Answer from the drawing. Dimensions are ordinates in mm from the lowest x, y and z of the part. Give positions to 0.01 mm unless a question says otherwise; leave off trailing zeros. Write each loop counter-clockwise with the first axis right and the second up, starting at its lowest first coordinate (ties: lowest second). Pieces come first, ordered by that corner, then holes. Notation, with made-up numbers: M -16.5,-15.75 L 0.5,-15.75 A28 cw 0.5,5.25 Z; hole C -13,83 d6. An arc over 180 degrees is marked long. Write each question's results on one line, items separated by ' | '. Start each with the question number.
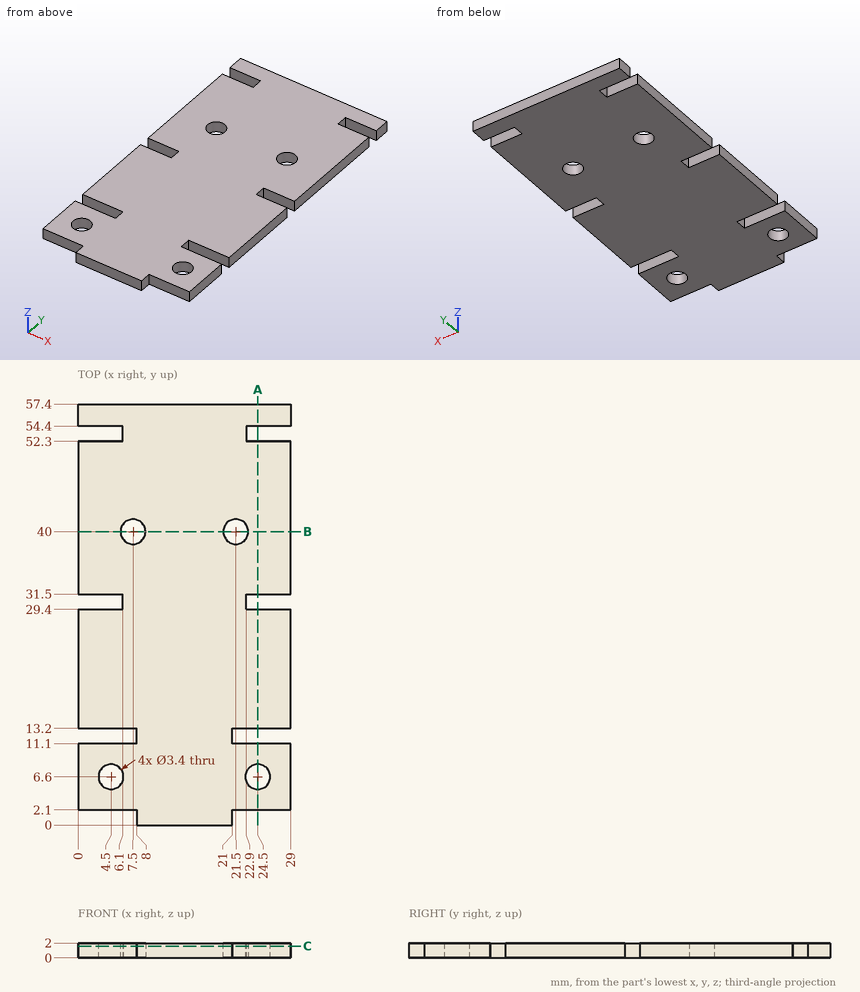
Item 1: Section C-C, the plane z = 1.6 is taken. Give the number of separate pieces and of enclosed holes in the cut face, then the cut area to 3 significant figures.
Item 2: Section B-B, the plane y = 40 is taken. Determine the outline of the cut face in (x, z).
Item 3: Straight lines are drawn through the part: line 1 (Y direction, x = 26.5, z = 1.4); line 2 (Y direction, x = 4.5, z = 0.5); line 3 (Y direction, x = 7.5, z = 1.4). For each, find the intervals that lie inside material, in ascending order.
Item 4: Section A-A, the plane x = 24.5 is taken. Determine the outline of the cut face in (y, z).
Item 5: Given P1, Ø2, axis at x = 4.5, y = 6.6, coming from the -Z side; P2, Ø1, axis at y = 53, z = 1, coming from the -X side; P3, Ø1, axis at x = 23.5, z = 1, coming from the -Y side, each flat-ended and moving along its own axis, determine where each tip first touches the part or whether it passes through.
Worked out:
1) separate pieces: 1 | enclosed holes: 4 | area: 1,510 mm²
2) outline: M 0,0 L 5.8,0 L 5.8,2 L 0,2 Z; M 9.2,0 L 19.8,0 L 19.8,2 L 9.2,2 Z; M 23.2,0 L 29,0 L 29,2 L 23.2,2 Z
3) line 1: y = 2.1 to 11.1, 13.2 to 29.4, 31.5 to 52.3, 54.4 to 57.4 | line 2: y = 2.1 to 4.9, 8.3 to 11.1, 13.2 to 29.4, 31.5 to 52.3, 54.4 to 57.4 | line 3: y = 2.1 to 11.1, 13.2 to 38.3, 41.7 to 57.4
4) outline: M 2.1,0 L 4.9,0 L 4.9,2 L 2.1,2 Z; M 8.3,0 L 11.1,0 L 11.1,2 L 8.3,2 Z; M 13.2,0 L 29.4,0 L 29.4,2 L 13.2,2 Z; M 31.5,0 L 52.3,0 L 52.3,2 L 31.5,2 Z; M 54.4,0 L 57.4,0 L 57.4,2 L 54.4,2 Z
5) P1: passes through | P2: stops at x = 6.1 | P3: stops at y = 2.1
